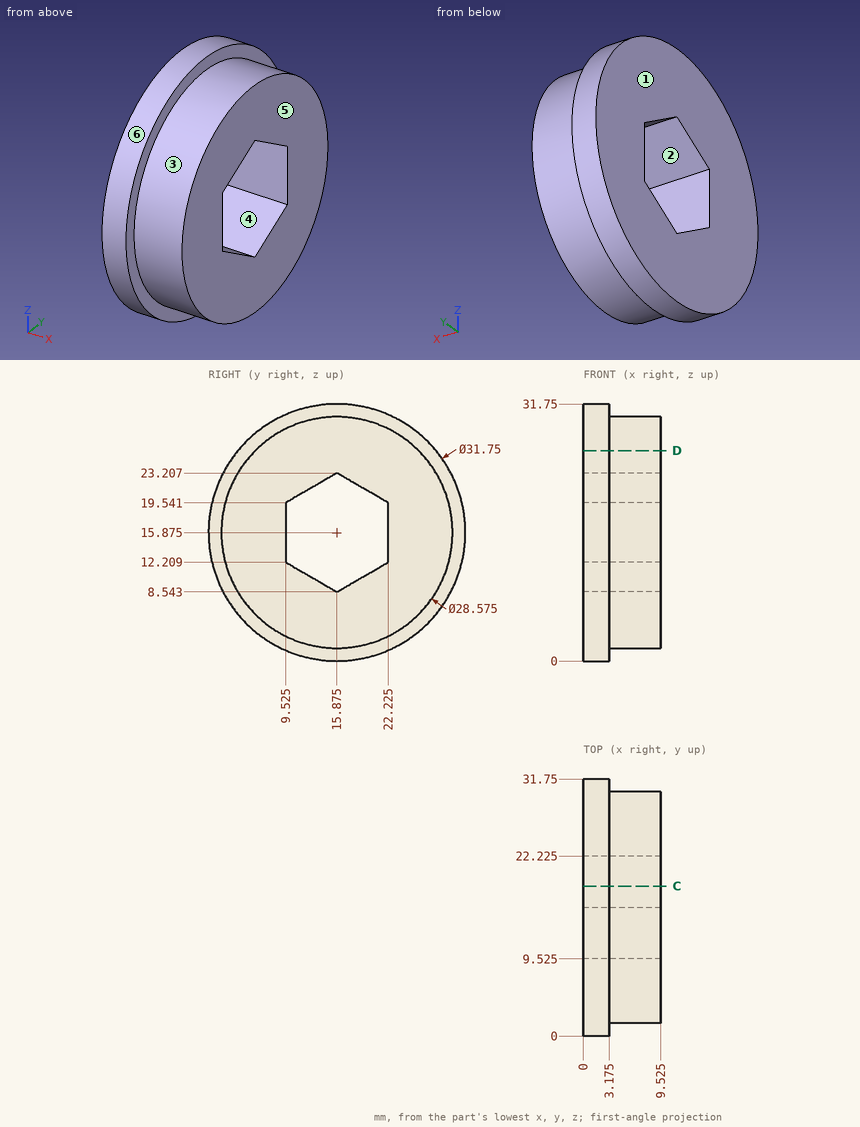
Print and shaded views of the part. All mm, measured from the part's lowest x, y and z. A direction names the side the tool comes from. Coordinates: 2 decimals unless noted, no trailing zeros. Order: outer loops, then holes, each group sorted by start corner. A loop starts at its lowest first (then second) coordinate and runs counter-clockwise, first axis right, second up. Notation, with made-up numbers: M -39,61.25 L -30,61.25 A15 cw -30,77.25 Z; hole C -11.5,-36.5 d6. An arc over 180 degrees is marked long. Write each question's results on one line, items separated by ' | '. Start each with the question number.
Q1. Cut at C-C (y = 18.5). List the corners of the cut face in (x, z) (1 decimal).
Q2. Which spindle directions (+Z, -Z, +X, -X, +Y, -Y) get a long thin tool onto all of the face, cutting with end or side? Do the marked faces 1, 2 and 3. Say none if no direction does.
Q3. Flat gauge pins, fed straight in: P1, Ø5, axis at x = 3, y = 20.5, coming from the +Z side; P2, Ø5, axis at x = 4.5, z = 10.5, coming from the +Y side; P3, Ø2, axis at x = 3.5, y = 26.5, coming from the -Z side. Where does each tip first touch, or does it go through?
Q4. Pull direction Z, two halves, no side cores. Call the marked faces 4, 5 and 6: +Z half, -Z half, draft (parallel to the pull), parting line (faces both ways), or undercut.
Q5. Drill centre lines: probe 1 along Z at (x, y) = (7.75, 18) (1 decimal); probe 2 along Y at (x, z) = (3.5, 15) (1 decimal); probe 3 along Y at (x, z) = (5.75, 14) (1 decimal). Where is each one in solid material? Low to high. Write a range as from..to.
Q6. Cut at D-D (z = 26). List the corners of the cut face in (x, y) (1 decimal).
Found:
1) outline: M 0,0.2 L 3.2,0.2 L 3.2,1.8 L 9.5,1.8 L 9.5,10.1 L 0,10.1 Z; M 0,21.7 L 9.5,21.7 L 9.5,29.9 L 3.2,29.9 L 3.2,31.5 L 0,31.5 Z
2) face 1: +Z, -Z, -X, +Y, -Y | face 2: +X, -X | face 3: +X
3) P1: z = 31.61 | P2: y = 31.41 | P3: z = 3.29
4) face 4: undercut | face 5: draft | face 6: parting line
5) probe 1: 1.7..9.8, 22..30 | probe 2: 1.6..9.5, 22.2..30.1 | probe 3: 1.7..9.5, 22.2..30
6) outline: M 0,3.6 L 3.2,3.6 L 3.2,5.8 L 9.5,5.8 L 9.5,26 L 3.2,26 L 3.2,28.1 L 0,28.1 Z
